from build123d import *

# Parameters (mm, degrees)
F0_W           = 51.3226017356
F0_H           = 45.5124992877
F1_DEPTH       = 25.4
F2_T           = -2.54
F3_R           = 5.08
F4_W           = 46.2916959077
F4_H           = 2.1475534886
F5_DEPTH       = 23.114
F5_DEPTH_BACK  = 18.034
F6_R           = 6.2989363063
F7_DEPTH       = 25.4
F7_DEPTH_BACK  = 36.83
F8_R           = 4.4507292133
F9_DEPTH       = 35.56
F9_DEPTH_BACK  = 25.4
F10_R          = 3.3711078554
F11_DEPTH      = 27.686
F11_DEPTH_BACK = 52.2224
F12_T4_DEPTH   = 70.9124992877
F12_T10_DEPTH  = 70.9124992877
F12_T16_DEPTH  = 70.9124992877
F12_T23_DEPTH  = 70.9124992877
F12_T29_DEPTH  = 70.9124992877
F12_T35_DEPTH  = 70.9124992877
F12_T41_DEPTH  = 70.9124992877
F12_T47_DEPTH  = 70.9124992877
F12_T54_DEPTH  = 70.9124992877
F12_T60_DEPTH  = 70.9124992877


# Not quite as in the source:
# - a fillet or chamfer that OpenCascade refuses, or shapes differently, is made with other operations: its cross-section is extruded or revolved along the edge and cut away or added


with BuildPart() as f1:
    # F0 (on Top) → F1 (new body)
    with BuildSketch(Plane.XY):
        with Locations((-0.7262639701, -2.4208771065)):
            Rectangle(F0_W, F0_H)
    extrude(amount=F1_DEPTH)

    # F2
    f2_openings = [f1.faces().sort_by_distance(p)[0] for p in [
        (-0.726264, -2.420877, 25.4),
    ]]
    offset(amount=F2_T, openings=f2_openings)

    # F3
    f3_edges = [f1.edges().sort_by_distance(p)[0] for p in [
        (-0.726264, -25.177127, 0),
        (-26.387565, -2.420877, 0),
        (-0.726264, 17.795373, 2.54),
        (22.395037, -2.420877, 2.54),
        (-0.726264, 20.335373, 0),
        (24.935037, -2.420877, 0),
    ]]
    fillet(f3_edges, radius=F3_R)

    # F4 (on Front) → F5 (join, two sides)
    with BuildSketch(Plane.XZ) as f5_sk:
        with Locations((-0.7661757991, 24.4599720463)):
            Rectangle(F4_W, F4_H)
    extrude(amount=F5_DEPTH)
    extrude(f5_sk.sketch, amount=-F5_DEPTH_BACK)

    # F6 (on Top) → F7 (cut, two sides)
    with BuildSketch(Plane.XY) as f7_sk:
        with Locations((-8.230984211, 5.3259306587)):
            Circle(F6_R)
    extrude(amount=F7_DEPTH, mode=Mode.SUBTRACT)
    extrude(f7_sk.sketch, amount=-F7_DEPTH_BACK, mode=Mode.SUBTRACT)

    # F8 (on Top) → F9 (join, two sides)
    with BuildSketch(Plane.XY) as f9_sk:
        with Locations((4.1154921055, -5.0838431343)):
            Circle(F8_R)
    extrude(amount=F9_DEPTH)
    extrude(f9_sk.sketch, amount=-F9_DEPTH_BACK)

    # F10 (on Top) → F11 (cut, two sides)
    with BuildSketch(Plane.XY) as f11_sk:
        with Locations((4.1154921055, -5.0838431343)):
            Circle(F10_R)
    extrude(amount=-F11_DEPTH, mode=Mode.SUBTRACT)
    extrude(f11_sk.sketch, amount=F11_DEPTH_BACK, mode=Mode.SUBTRACT)

    # F12: fillet of radius 5.08 on 2 edges, made by hand


with BuildPart() as f12_tool2:
    # F12_s3 → F12_t4 (new body)
    with BuildSketch(Plane.XZ.offset(37.8771267503)):
        with BuildLine():
            ThreePointArc((24.9350368977, 20.32), (23.4471393461, 23.9121024484), (19.8550368977, 25.4))
            Line((19.8550368977, 25.4), (24.9350368977, 25.4))
            Line((24.9350368977, 25.4), (24.9350368977, 20.32))
        make_face()
    extrude(amount=-F12_T4_DEPTH)

    split(bisect_by=Plane.YZ.offset(22.3796721548), keep=Keep.TOP)

    split(bisect_by=Plane.XZ.offset(23.114), keep=Keep.TOP)


with BuildPart() as f1_1:
    add(f1.part)

    # F12_t1: cut F12_tool2
    add(f12_tool2.part, mode=Mode.SUBTRACT)


with BuildPart() as f12_tool8:
    # F12_s9 → F12_t10 (new body)
    with BuildSketch(Plane.XZ.offset(37.8771267503)):
        with BuildLine():
            ThreePointArc((24.9350368977, 20.32), (23.4471393461, 23.9121024484), (19.8550368977, 25.4))
            Line((19.8550368977, 25.4), (24.9350368977, 25.4))
            Line((24.9350368977, 25.4), (24.9350368977, 20.32))
        make_face()
    extrude(amount=-F12_T10_DEPTH)

    split(bisect_by=Plane.YZ.offset(22.3796721548), keep=Keep.BOTTOM)

    split(bisect_by=Plane.XZ.offset(23.114), keep=Keep.TOP)


with BuildPart() as f1_2:
    add(f1_1.part)

    # F12_t7: cut F12_tool8
    add(f12_tool8.part, mode=Mode.SUBTRACT)


with BuildPart() as f12_tool14:
    # F12_s15 → F12_t16 (new body)
    with BuildSketch(Plane.XZ.offset(37.8771267503)):
        with BuildLine():
            ThreePointArc((24.9350368977, 20.32), (23.4471393461, 23.9121024484), (19.8550368977, 25.4))
            Line((19.8550368977, 25.4), (24.9350368977, 25.4))
            Line((24.9350368977, 25.4), (24.9350368977, 20.32))
        make_face()
    extrude(amount=-F12_T16_DEPTH)

    split(bisect_by=Plane.YZ.offset(22.3796721548), keep=Keep.TOP)

    split(bisect_by=Plane.XZ.offset(-18.034), keep=Keep.TOP)

    split(bisect_by=Plane.XZ.offset(23.114), keep=Keep.BOTTOM)


with BuildPart() as f1_3:
    add(f1_2.part)

    # F12_t13: cut F12_tool14
    add(f12_tool14.part, mode=Mode.SUBTRACT)


with BuildPart() as f12_tool21:
    # F12_s22 → F12_t23 (new body)
    with BuildSketch(Plane.XZ.offset(37.8771267503)):
        with BuildLine():
            ThreePointArc((24.9350368977, 20.32), (23.4471393461, 23.9121024484), (19.8550368977, 25.4))
            Line((19.8550368977, 25.4), (24.9350368977, 25.4))
            Line((24.9350368977, 25.4), (24.9350368977, 20.32))
        make_face()
    extrude(amount=-F12_T23_DEPTH)

    split(bisect_by=Plane.YZ.offset(22.3796721548), keep=Keep.TOP)

    split(bisect_by=Plane.XZ.offset(-18.034), keep=Keep.BOTTOM)


with BuildPart() as f1_4:
    add(f1_3.part)

    # F12_t20: cut F12_tool21
    add(f12_tool21.part, mode=Mode.SUBTRACT)


with BuildPart() as f12_tool27:
    # F12_s28 → F12_t29 (new body)
    with BuildSketch(Plane.XZ.offset(37.8771267503)):
        with BuildLine():
            ThreePointArc((24.9350368977, 20.32), (23.4471393461, 23.9121024484), (19.8550368977, 25.4))
            Line((19.8550368977, 25.4), (24.9350368977, 25.4))
            Line((24.9350368977, 25.4), (24.9350368977, 20.32))
        make_face()
    extrude(amount=-F12_T29_DEPTH)

    split(bisect_by=Plane.YZ.offset(22.3796721548), keep=Keep.BOTTOM)

    split(bisect_by=Plane.XZ.offset(-18.034), keep=Keep.BOTTOM)


with BuildPart() as f1_5:
    add(f1_4.part)

    # F12_t26: cut F12_tool27
    add(f12_tool27.part, mode=Mode.SUBTRACT)


with BuildPart() as f12_tool33:
    # F12_s34 → F12_t35 (new body)
    with BuildSketch(Plane.XZ.offset(-33.0353725374)):
        with BuildLine():
            ThreePointArc((-21.3075648379, 25.4), (-24.8996672864, 23.9121024484), (-26.3875648379, 20.32))
            Line((-26.3875648379, 20.32), (-26.3875648379, 25.4))
            Line((-26.3875648379, 25.4), (-21.3075648379, 25.4))
        make_face()
    extrude(amount=F12_T35_DEPTH)

    split(bisect_by=Plane.XZ.offset(-18.034), keep=Keep.BOTTOM)

    split(bisect_by=Plane.YZ.offset(-23.9120237529), keep=Keep.TOP)


with BuildPart() as f1_6:
    add(f1_5.part)

    # F12_t32: cut F12_tool33
    add(f12_tool33.part, mode=Mode.SUBTRACT)


with BuildPart() as f12_tool39:
    # F12_s40 → F12_t41 (new body)
    with BuildSketch(Plane.XZ.offset(-33.0353725374)):
        with BuildLine():
            ThreePointArc((-21.3075648379, 25.4), (-24.8996672864, 23.9121024484), (-26.3875648379, 20.32))
            Line((-26.3875648379, 20.32), (-26.3875648379, 25.4))
            Line((-26.3875648379, 25.4), (-21.3075648379, 25.4))
        make_face()
    extrude(amount=F12_T41_DEPTH)

    split(bisect_by=Plane.XZ.offset(-18.034), keep=Keep.BOTTOM)

    split(bisect_by=Plane.YZ.offset(-23.9120237529), keep=Keep.BOTTOM)


with BuildPart() as f1_7:
    add(f1_6.part)

    # F12_t38: cut F12_tool39
    add(f12_tool39.part, mode=Mode.SUBTRACT)


with BuildPart() as f12_tool45:
    # F12_s46 → F12_t47 (new body)
    with BuildSketch(Plane.XZ.offset(-33.0353725374)):
        with BuildLine():
            ThreePointArc((-21.3075648379, 25.4), (-24.8996672864, 23.9121024484), (-26.3875648379, 20.32))
            Line((-26.3875648379, 20.32), (-26.3875648379, 25.4))
            Line((-26.3875648379, 25.4), (-21.3075648379, 25.4))
        make_face()
    extrude(amount=F12_T47_DEPTH)

    split(bisect_by=Plane.XZ.offset(-18.034), keep=Keep.TOP)

    split(bisect_by=Plane.YZ.offset(-23.9120237529), keep=Keep.BOTTOM)

    split(bisect_by=Plane.XZ.offset(23.114), keep=Keep.BOTTOM)


with BuildPart() as f1_8:
    add(f1_7.part)

    # F12_t44: cut F12_tool45
    add(f12_tool45.part, mode=Mode.SUBTRACT)


with BuildPart() as f12_tool52:
    # F12_s53 → F12_t54 (new body)
    with BuildSketch(Plane.XZ.offset(-33.0353725374)):
        with BuildLine():
            ThreePointArc((-21.3075648379, 25.4), (-24.8996672864, 23.9121024484), (-26.3875648379, 20.32))
            Line((-26.3875648379, 20.32), (-26.3875648379, 25.4))
            Line((-26.3875648379, 25.4), (-21.3075648379, 25.4))
        make_face()
    extrude(amount=F12_T54_DEPTH)

    split(bisect_by=Plane.YZ.offset(-23.9120237529), keep=Keep.TOP)

    split(bisect_by=Plane.XZ.offset(23.114), keep=Keep.TOP)


with BuildPart() as f1_9:
    add(f1_8.part)

    # F12_t51: cut F12_tool52
    add(f12_tool52.part, mode=Mode.SUBTRACT)


with BuildPart() as f12_tool58:
    # F12_s59 → F12_t60 (new body)
    with BuildSketch(Plane.XZ.offset(-33.0353725374)):
        with BuildLine():
            ThreePointArc((-21.3075648379, 25.4), (-24.8996672864, 23.9121024484), (-26.3875648379, 20.32))
            Line((-26.3875648379, 20.32), (-26.3875648379, 25.4))
            Line((-26.3875648379, 25.4), (-21.3075648379, 25.4))
        make_face()
    extrude(amount=F12_T60_DEPTH)

    split(bisect_by=Plane.YZ.offset(-23.9120237529), keep=Keep.BOTTOM)

    split(bisect_by=Plane.XZ.offset(23.114), keep=Keep.TOP)


with BuildPart() as f1_10:
    add(f1_9.part)

    # F12_t57: cut F12_tool58
    add(f12_tool58.part, mode=Mode.SUBTRACT)


solid = f1_10.part
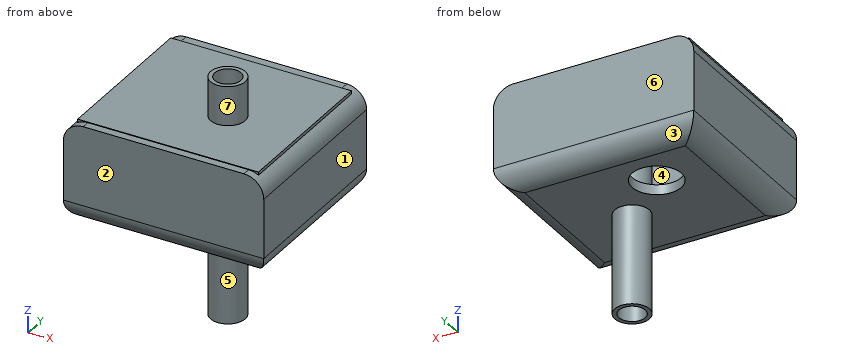
Part model, mm, in its own coordinate system. Face numbers are marked on the shaded views. A direction names the side the tool comes from. Round coordinates to 2 decimals unless told otherwise and drop trailing zeros. Write each loop counter-clockwise with the first axis right and the second up, starting at its lowest first coordinate (ties: lowest second). Pieces come first, ordered by that corner, then holes. Notation, with made-up numbers: (83.25, 77.25) - (141.25, 77.25) arc R8 ccw to (141.25, 83.25) - close; hole circle Ø5 at (-12, 16.25). An arc over 180 degrees is marked (long way). Use CSV: the item, a comma, the result in double quotes.
Item 1: Flat gauge pins, fed straight in: P1, Ø12, axis at x = 2.5, y = -20, coming from the +Z side; P2, Ø17.5, axis at x = -8, y = 3.5, coming from the -Z side; P3, Ø0.7, axis at x = -4, y = 18.5, coming from the +Z side; P4, Ø1.5, axis at y = -12, z = -19, coming from the -X side. Where does each tip first touch, or does it go through?
Results list:
P1,"stops at z = 25.53"
P2,"stops at z = 0"
P3,"stops at z = 25.4"
P4,"passes through"
Item 2: Slice it at A-A, the plane x = 12.5. Write the cut outline in (y, z).
Results list:
outline,"(-25.18, 5.08) arc R5.08 ccw to (-20.1, 0) - (15.26, 0) arc R5.08 ccw to (20.34, 5.08) - (20.34, 25.4) - (18.03, 25.4) - (18.03, 25.53) - (-23.11, 25.53) - (-23.11, 25.4) - (-25.18, 25.4) - close; hole (-22.64, 2.54) - (12.72, 2.54) arc R5.08 ccw to (17.8, 7.62) - (17.8, 23.39) - (-22.64, 23.39) - close"
Item 3: Slice it at B-B, the plane y = -6. Count the separate pieces of the cut face and the enclosed holes in it, then the cut area to 3 significant figures.
Results list:
separate pieces,"2"
enclosed holes,"1"
area,"425 mm²"
Item 4: Pull direction Y, two halves, no side cores. Call the marked faces 1, 2, 3 and 4: pulls with the +Y half, pulls with the -Y half, needs draft (parallel to the pull), parting line crosses it, or undercut.
Results list:
face 1,"needs draft"
face 2,"pulls with the -Y half"
face 3,"pulls with the +Y half"
face 4,"undercut"
Item 5: Tool access for the marked faces 5, 6 and 7: list every direction of +Z, -Z, +X, -X, +Y, -Y with a clear straight run to the whole face (end or side of a thin tool).
Results list:
face 5,"-Z"
face 6,"+Z, -Z, +X, -X, +Y"
face 7,"+Z"
Item 6: Slice it at D-D, the plane y = -15.5. Write the cut outline in (x, z), then the cut area to 3 significant figures.
Results list:
outline,"(-26.39, 5.08) arc R5.08 ccw to (-21.31, 0) - (19.86, 0) arc R5.08 ccw to (24.94, 5.08) - (24.94, 20.32) arc R5.08 ccw to (22.4, 24.72) - (22.4, 7.62) arc R5.08 cw to (17.32, 2.54) - (-23.85, 2.54) - (-23.85, 23.39) - (22.38, 23.39) - (22.38, 25.53) - (-23.91, 25.53) - (-23.91, 24.68) arc R5.08 ccw to (-26.39, 20.32) - close"
area,"330 mm²"
Item 7: Wall check: L1, parallel to Z at x = -15.5, y = -19; L2, parallel to Y at x = 8, z = 19; L3, parallel to Y at x = -17.5, z = 10. Give the ranges that are in metal, low to high.
Results list:
L1,"z = 0 to 2.54, 23.39 to 25.53"
L2,"y = -25.18 to -22.64, -7.26 to -2.91, 17.8 to 20.34"
L3,"y = -25.18 to -22.64, 17.8 to 20.34"
Item 8: Slice it at C-C, the plane z = 12.5. Write the cut outline in (x, y).
Results list:
outline,"(-26.39, -25.18) - (24.94, -25.18) - (24.94, 20.34) - (-26.39, 20.34) - close; circle Ø8.9 at (4.12, -5.08); hole (-23.85, -22.64) - (22.4, -22.64) - (22.4, 17.8) - (-23.85, 17.8) - close; hole circle Ø6.74 at (4.12, -5.08)"
